The listing builds one solid part. Answer for the finished solid, in the listing's coordinates (mm). Face numbers are marked on the shaded views. Round coordinates to 2 decimals unless told otherwise and drop trailing zeros.
(1) Find the intervals of material crossed by probe 1 along X at (y, z) = (5.25, 3.25); probe 2 along X at (y, z) = (5.25, -3.75); probe 3 along X at (y, z) = (6.25, 7.5), in increasing order.
(2) The mould has two halves that part along X. Classify the marked faces 1, 2 and 3: +X half, -X half, draft (parallel to the pull), parting line (faces both ways), or undercut.
(3) Each of these flat-tipped pins is pushed along its axis until it touches: pin 1 Ø3 at (x, y) = (-39, 2) entering from +Z; pin 2 Ø4 at (x, y) = (-37, 6) entering from +Z; pin 3 Ø4 at (y, z) = (4, 11) entering from -X; pin 4 Ø5 at (x, z) = (-26, 15.5) entering from -Y. Where does it stop, or does it pass through?
from build123d import *

# Parameters (mm, degrees)
BOSS_EXTRUDE1_DEPTH = 9.525
SKETCH3_R           = 2
CUT_EXTRUDE1_DEPTH  = 2.7
SKETCH4_R           = 1
CUT_EXTRUDE2_DEPTH  = 51.984772229
FILLET2_R           = 4.7625
FILLET3_R           = 0.762


with BuildPart() as part:
    # Sketch1 → Boss-Extrude1 (new body)
    with BuildSketch(Plane(origin=(0, 0, 0), x_dir=(1, 0, 0), z_dir=(0, 1, 0))):
        Polygon((-27.422743224, -19.119856123), (-46.29298428, -16.509012872), (-42.811859946, 8.651308536), (-23.941618889, 6.040465285), align=None)
    extrude(amount=BOSS_EXTRUDE1_DEPTH)

    # Sketch3 → Cut-Extrude1 (cut)
    with BuildSketch(Plane(origin=(0.316670388, 0, -2.684144047), x_dir=(-0.9905638349724136, 0, -0.13705213914691383), z_dir=(0.13705213914691383, 0, -0.9905638349724136))):
        with Locations((40.495544979, 4.7625)):
            Circle(SKETCH3_R)
    extrude(amount=-CUT_EXTRUDE1_DEPTH, mode=Mode.SUBTRACT)

    # Sketch4 → Cut-Extrude2 (cut, through all)
    with BuildSketch(Plane(origin=(0.000303759, 0, -0.00219546), x_dir=(-0.9905638349724136, 0, -0.13705213914691383), z_dir=(0.1370521391469138, 0, -0.9905638349724135))):
        with Locations((40.549730429, 4.7625)):
            Circle(SKETCH4_R)
    extrude(amount=-CUT_EXTRUDE2_DEPTH, mode=Mode.SUBTRACT)

    # Fillet2
    fillet2_edges = [part.edges().sort_by_distance(p)[0] for p in [
        (-44.552422113, 0, 3.928852168),
        (-44.552422113, 9.525, 3.928852168),
    ]]
    fillet(fillet2_edges, radius=FILLET2_R - 0.0001)  # a hair under: the kernel refuses the full size

    # Fillet3
    fillet3_edges = [part.edges().sort_by_distance(p)[0] for p in [
        (-34.499133148, 9.525, 18.140783052),
        (-34.499133148, 0, 18.140783052),
        (-44.911271882, 1.394874665, 16.700183429),
        (-44.911271882, 8.130125335, 16.700183429),
        (-41.430147548, 1.394874665, -8.460137979),
        (-41.430147548, 8.130125335, -8.460137979),
        (-31.018008814, 0, -7.019538357),
        (-31.018008814, 9.525, -7.019538357),
    ]]
    fillet(fillet3_edges, radius=FILLET3_R)


solid = part.part
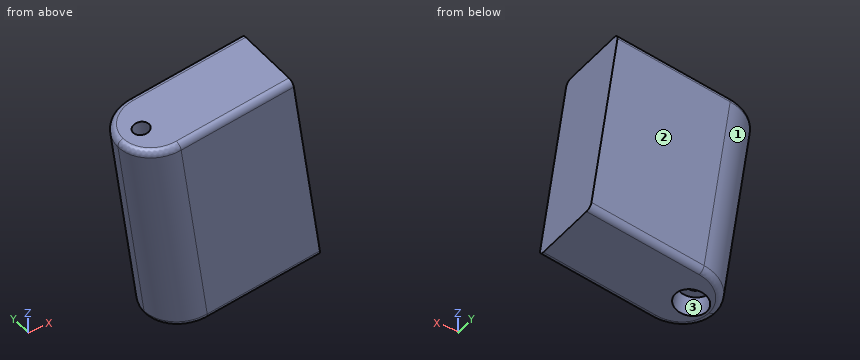
Solutions:
1. probe 1: x = -44.43 to -42.27, -40.5 to -25.23
1. probe 2: x = -43.46 to -41.3, -39.54 to -24.26
1. probe 3: x = -44.81 to -25.82
2. face 1: -X half
2. face 2: draft
2. face 3: undercut
3. pin 1: stops at z = 17.73
3. pin 2: stops at z = 18.07
3. pin 3: stops at x = -45.79
3. pin 4: stops at y = 0
